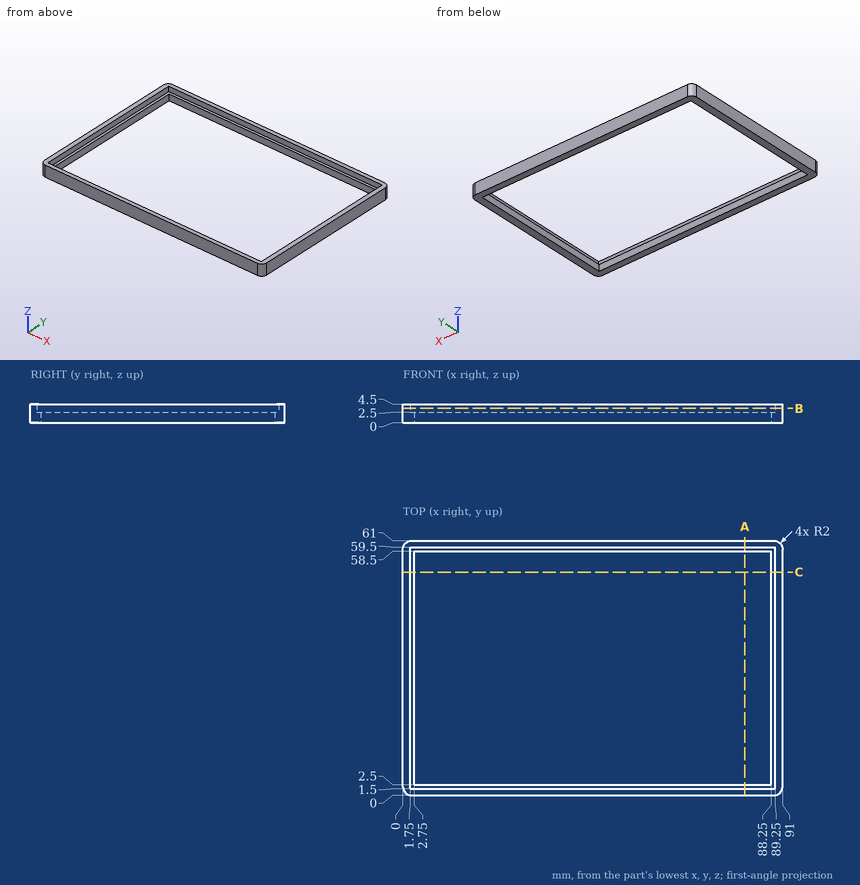
Design review of the part shown in the three views and the two pictorial views. Dimensions are in mm from the part's minimum x, y and z. Round coordinates to 2 decimals unless told otherwise and drop trailing zeros. Order: outer loops, then holes, each group sorted by start corner. A loop starts at its lowest first (then second) coordinate and runs counter-clockwise, first axis right, second up.
(1) Wall thickness on L1, parallel to Y at x = 14.5, z = 3; L2, parallel to X at y = 39, z = 2.9; L3, parallel to Y at x = 73, z = 0.7: over which ranges is each line inside the solid? List them lowest first.
Working result:
L1: y = 0 to 1.5, 59.5 to 61
L2: x = 0 to 1.75, 89.25 to 91
L3: y = 0 to 2.5, 58.5 to 61
(2) Take a section at B-B, the plane z = 3.45. State the section outline as (x, y) points, plus the area to 3 significant figures.
Working result:
outline: (0, 2) arc R2 ccw to (2, 0) - (89, 0) arc R2 ccw to (91, 2) - (91, 59) arc R2 ccw to (89, 61) - (2, 61) arc R2 ccw to (0, 59) - close; hole (1.75, 1.5) - (89.25, 1.5) - (89.25, 59.5) - (1.75, 59.5) - close
area: 473 mm2
(3) Take a section at C-C, the plane y = 53.5. State the section outline as (x, z) points, plus the area to 4 significant figures.
Working result:
outline: (0, 0) - (2.75, 0) - (2.75, 2.5) - (1.75, 2.5) - (1.75, 4.5) - (0, 4.5) - close; (88.25, 0) - (91, 0) - (91, 4.5) - (89.25, 4.5) - (89.25, 2.5) - (88.25, 2.5) - close
area: 20.75 mm2
(4) For P1, Ø17.5, axis at x = 52.5, y = 17.5, coming from the +Z side, flat-tipped, find the tip position at first contact; note if it passes through.
Working result:
P1: passes through
(5) Take a section at A-A, the plane x = 82. State the section outline as (y, z) points, plus the area to 3 significant figures.
Working result:
outline: (0, 0) - (2.5, 0) - (2.5, 2.5) - (1.5, 2.5) - (1.5, 4.5) - (0, 4.5) - close; (58.5, 0) - (61, 0) - (61, 4.5) - (59.5, 4.5) - (59.5, 2.5) - (58.5, 2.5) - close
area: 18.5 mm2
